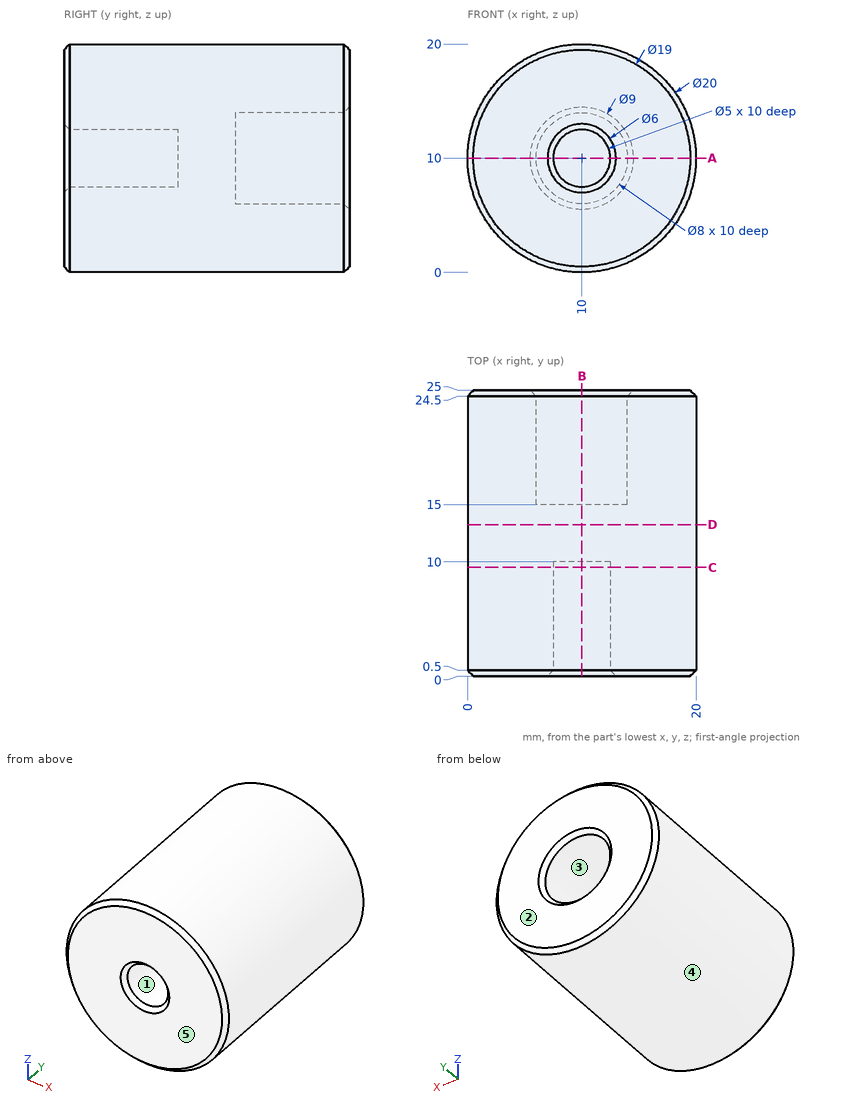
Print and shaded views of the part. All mm, measured from the part's lowest x, y and z. A direction names the side the tool comes from. Give positions to 0.01 mm unless a question says otherwise; leave off trailing zeros. Loops run counter-clockwise (first coordinate to the right, second up) from the corner with the lowest first, then second, coordinate; pieces in that order, holes last. Notation, with made-up numbers: (57, -17) - (77, -17) arc R29 ccw to (77, 10) - close; hole circle Ø1 at (-0.75, -8.75). An arc over 180 degrees is marked (long way). Use a Markdown table: item, result.
(1) Band-saw the part on A-A (z = 10). Give the cut face in (x, y).
Taken from the geometry:
| item | result |
|---|---|
| outline | (0, 0.5) - (0.5, 0) - (7, 0) - (7.5, 0.5) - (7.5, 10) - (12.5, 10) - (12.5, 0.5) - (13, 0) - (19.5, 0) - (20, 0.5) - (20, 24.5) - (19.5, 25) - (14.5, 25) - (14, 24.5) - (14, 15) - (6, 15) - (6, 24.5) - (5.5, 25) - (0.5, 25) - (0, 24.5) - close |
(2) Pull direction X, two halves, no side cores. Call the marked faces 3, 4 and 5: +X half, -X half, draft (parallel to the pull), parting line (faces both ways), or undercut.
Taken from the geometry:
| item | result |
|---|---|
| face 3 | undercut |
| face 4 | parting line |
| face 5 | draft |
(3) Which spindle directions (+Z, -Z, +X, -X, +Y, -Y) get a long thin tool onto all of the face, cutting with end or side? Do the marked faces 1 and 2. Say none if no direction does.
Taken from the geometry:
| item | result |
|---|---|
| face 1 | -Y |
| face 2 | +Z, -Z, +X, -X, +Y |
(4) Band-saw the part on B-B (x = 10). Give the cut face in (y, z), and give its area (3 significant figures).
Taken from the geometry:
| item | result |
|---|---|
| outline | (0, 0.5) - (0.5, 0) - (24.5, 0) - (25, 0.5) - (25, 5.5) - (24.5, 6) - (15, 6) - (15, 14) - (24.5, 14) - (25, 14.5) - (25, 19.5) - (24.5, 20) - (0.5, 20) - (0, 19.5) - (0, 13) - (0.5, 12.5) - (10, 12.5) - (10, 7.5) - (0.5, 7.5) - (0, 7) - close |
| area | 369 mm2 |
(5) Band-saw the part on D-D (y = 13.25). Give the cut face in (x, z), and give its area (3 significant figures).
Taken from the geometry:
| item | result |
|---|---|
| outline | circle Ø20 at (10, 10) |
| area | 314 mm2 |
(6) Band-saw the part on C-C (y = 9.5). Give the cut face in (x, z).
Taken from the geometry:
| item | result |
|---|---|
| outline | circle Ø20 at (10, 10); hole circle Ø5 at (10, 10) |
(7) Wall check: line 1 along X through (y, z) = (19.5, 10); line 2 along X through (y, z) = (1.75, 10); line 3 along Z through (x, y) = (9.75, 14). Give the ranges that are in metal, low to high.
Taken from the geometry:
| item | result |
|---|---|
| line 1 | 0 to 6, 14 to 20 |
| line 2 | 0 to 7.5, 12.5 to 20 |
| line 3 | 0 to 20 |
(8) Drop flat-ended pins along their axis: pin 1 Ø1.5 at (y, z) = (20.5, 5) entering from +X; pin 2 Ø2 at (x, y) = (7, 16.5) entering from -Z; pin 3 Ø3 at (x, z) = (10, 10) entering from -Y. Give the stop position or say it passes through.
Taken from the geometry:
| item | result |
|---|---|
| pin 1 | x = 19.05 |
| pin 2 | z = 0.2 |
| pin 3 | y = 10 |
